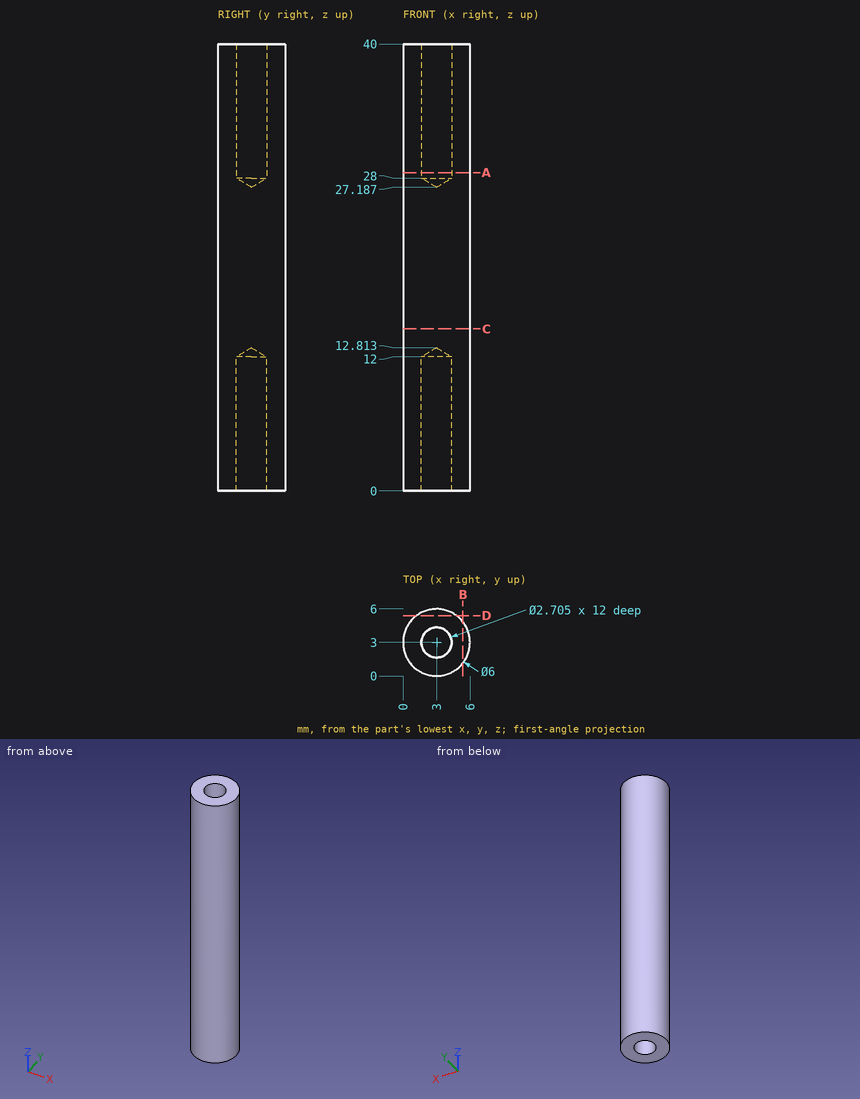
Input: dimensioned drawing with shaded views. Units: mm. Origin: part minimum x, y, z. Round coordinates to 2 decimals unless told otherwise and drop trailing zeros. Order: outer loops, then holes, each group sorted by start corner. A loop starts at its lowest first (then second) coordinate and runs counter-clockwise, first axis right, second up. Notation, with made-up numbers: (52.25, 45) -> (64.25, 45) arc R26 cw to (64.25, 70) -> close; hole circle Ø10 at (-40, -22.5). An arc over 180 degrees is marked (long way). One line per item, written item: value. Start each with the question number.
Q1. Section query C-C (z = 14.5). Return the cut outline in (x, y).
Q2. Section query A-A (z = 28.5). Return the cut outline in (x, y) (1 decimal).
Q3. Section query D-D (y = 5.4). Return the cut outline in (x, z).
Q4. Pin query (flat end, axial travel): pin 1 (1.5 mm diameter, centred on y = 2, z = 12.5, fed in from +X). Return the tip coordinate at first contact, or that it passes through.
Q5. Material intervals for probe 1 along Y at (x, z) = (3, 9.75); probe 2 along Y at (x, z) = (0.4, 3.5) (1 decimal); probe 3 along Y at (x, z) = (4.05, 30), sorted ascending.
Q6. Section query B-B (x = 5.35). Return the cut outline in (y, z) (1 decimal).
Findings below:
1. outline: circle Ø6 at (3, 3)
2. outline: circle Ø6 at (3, 3); hole circle Ø2.7 at (3, 3)
3. outline: (1.2, 0) -> (4.8, 0) -> (4.8, 40) -> (1.2, 40) -> close
4. pin 1: x = 5.99
5. probe 1: 0 to 1.65, 4.35 to 6
5. probe 2: 1.5 to 4.5
5. probe 3: 0.19 to 2.15, 3.85 to 5.81
6. outline: (1.1, 0) -> (4.9, 0) -> (4.9, 40) -> (1.1, 40) -> close
